from build123d import *

# Parameters (mm, degrees)
SKETCH1_W           = 4.2
SKETCH1_H           = 4.3
BOSS_EXTRUDE1_DEPTH = 7
FILLET1_R           = 1
FILLET2_R           = 3
FILLET3_R           = 1
SKETCH3_W           = 8
SKETCH3_H           = 7
BOSS_EXTRUDE2_DEPTH = 2
SKETCH2_R           = 1.4
CUT_EXTRUDE2_DEPTH  = 4
FILLET4_R           = 1


with BuildPart() as part:
    # Sketch1 → Boss-Extrude1 (new body)
    # profile 1 of 2: a face of its own
    with BuildSketch(Plane(origin=(0, 0, 0), x_dir=(1, 0, 0), z_dir=(0, 1, 0))):
        with BuildLine():
            ThreePointArc((7, 0), (-4.949747468, -4.949747468), (0, 7))
            Line((0, 7), (3.872983346, 7))
            Line((3.872983346, 7), (4, 7))
            Line((4, 7), (4, 14))
            Line((4, 14), (-4, 14))
            Line((-4, 14), (-4, 7))
            Line((-4, 7), (-3.872983346, 7))
            ThreePointArc((-3.872983346, 7), (-3.936655355, 6.964391188), (-4, 6.92820323))
            ThreePointArc((-4, 6.92820323), (-2.053343481, -7.73199719), (6.910323964, 4.030809189))
            Line((6.910323964, 4.030809189), (6.046533468, 3.52695804))
            ThreePointArc((6.046533468, 3.52695804), (6.757430513, 1.826782105), (7, 0))
        make_face()
        with Locations((0, 10.5)):
            Rectangle(SKETCH1_W, SKETCH1_H, mode=Mode.SUBTRACT)
    # profile 2 of 2: a face of its own
    with BuildSketch(Plane(origin=(0, 0, 0), x_dir=(1, 0, 0), z_dir=(0, 1, 0))):
        with BuildLine():
            Line((-4, 7), (-4, 6.92820323))
            ThreePointArc((-4, 6.92820323), (-3.936655355, 6.964391188), (-3.872983346, 7))
            Line((-3.872983346, 7), (-4, 7))
        make_face()
    extrude(amount=BOSS_EXTRUDE1_DEPTH)

    # Fillet1
    fillet1_edges = [part.edges().sort_by_distance(p)[0] for p in [
        (4, 3.5, -7),
        (-4, 3.5, -6.92820323),
    ]]
    fillet(fillet1_edges, radius=FILLET1_R)

    # Fillet2
    fillet2_edges = [part.edges().sort_by_distance(p)[0] for p in [
        (6.478428716, 0, -3.778883614),
        (6.478428716, 7, -3.778883614),
    ]]
    fillet(fillet2_edges, radius=FILLET2_R)

    # Fillet3
    fillet3_edges = [part.edges().sort_by_distance(p)[0] for p in [
        (0, 7, -8.35),
        (0, 0, -8.35),
    ]]
    fillet(fillet3_edges, radius=FILLET3_R)

    # Sketch3 → Boss-Extrude2 (add)
    with BuildSketch(Plane(origin=(0, 0, -14), x_dir=(-1, 0, 0), z_dir=(0, 0, -1))):
        with Locations((0, 3.5)):
            Rectangle(SKETCH3_W, SKETCH3_H)
    extrude(amount=BOSS_EXTRUDE2_DEPTH)

    # Sketch2 → Cut-Extrude2 (cut)
    with BuildSketch(Plane(origin=(0, 0, -16), x_dir=(-1, 0, 0), z_dir=(0, 0, -1))):
        with Locations((0, 3.5)):
            Circle(SKETCH2_R)
    extrude(amount=-CUT_EXTRUDE2_DEPTH, mode=Mode.SUBTRACT)

    # Fillet4
    fillet4_edges = [part.edges().sort_by_distance(p)[0] for p in [
        (4, 3.5, -16),
        (-4, 3.5, -16),
    ]]
    fillet(fillet4_edges, radius=FILLET4_R)


solid = part.part
Source: CAD feature listing. Evaluate the final solid. Frame: model axes, mm. A direction names the side the tool comes from. Give positions to 0.01 mm unless a question says otherwise; leave off trailing zeros. Write each loop counter-clockwise with the first axis right and the second up, starting at its lowest first coordinate (ties: lowest second). Pieces come first, ordered by that corner, then holes. Notation, with made-up numbers: (28, -31.5) -> (84, -31.5) arc R4 ccw to (84, -27.5) -> close; hole circle Ø4 at (-39.5, 64.25). An arc over 180 degrees is marked (long way). Return JSON: item names as keys, results as strings. Group by question number.
1. Material intervals for line 1 (Y direction, x = 0, z = -14.15); line 2 (X direction, y = 5, z = -11.25); line 3 (Z direction, x = 0, y = 3.25), sorted ascending. Write a range as from..to.
2. Section C-C, the plane z = 6. Output: boundary loops of the cut face in (x, y), then the cut area to 3 significant figures.
3. Access query for faces 1 (the face through (6.48, 3.49, -3.78)), 2 (the face through (3.715, 3.549, -7.301)), 3 (the face through (4, 3, -11)), 4 (the face through (0.303, 2.133, -14.348)). Directions: +Z, -Z, +X, -X, +Y, -Y. A direction counts if a zero-diameter tool reaches every point of the face in a straight line with its end or side. Return the directions, or none.
4. Pin query (flat end, axial travel): pin 1 Ø1 at (y, z) = (2.5, -8.5) entering from -X; pin 2 Ø0.9 at (x, y) = (2, 5) entering from +Z; pin 3 Ø2 at (y, z) = (2.5, -12.5) entering from +X. Return the tip coordinate at first contact, or that it passes through.
5. Section B-B, the plane y = 3.5. Output: boundary loops of the cut face in (x, z), then the cut area to 3 significant figures.
6. Section A-A, the plane x = -3.5. Output: boundary loops of the cut face in (y, z).
7. Section D-D, the plane x = 0.25. Output: boundary loops of the cut face in (y, z), then the cut area to 3 significant figures.
8. Mould query, pull axis Z, two halves, no side actions, for faces 5 (the face through (-2, 0, -7)), 6 (the face through (6.79, 6.14, -2.92)), 7 (the face through (0.029, 6.699, -8.065)). Classes: +Z half, -Z half, draft (parallel to the pull), parting line (faces both ways), or undercut.
Determined:
{
 "1": {"line 1": "y = 0..2.1, 4.9..7", "line 2": "x = -4..-2.1, 2.1..4", "line 3": "z = -8.35..-7, 7..8"},
 "2": {"outline": "(-5.29, 0) -> (-3.61, 0) -> (-3.61, 7) -> (-5.29, 7) -> close; (3.61, 0) -> (5.29, 0) -> (5.29, 7) -> (3.61, 7) -> close", "area": "23.6 mm2"},
 "3": {"face 1": "-Z, +Y, -Y", "face 2": "+X, +Y, -Y", "face 3": "-Z, +X, +Y, -Y", "face 4": "-Z"},
 "4": {"pin 1": "stops at x = -4", "pin 2": "stops at z = 7.85", "pin 3": "stops at x = 4"},
 "5": {"outline": "(-4.44, -6.65) arc R1 cw to (-4, -7.48) -> (-4, -15) arc R1 ccw to (-3, -16) -> (-1.4, -16) -> (-1.4, -12.65) -> (-2.1, -12.65) -> (-2.1, -8.35) -> (2.1, -8.35) -> (2.1, -12.65) -> (1.4, -12.65) -> (1.4, -16) -> (3, -16) arc R1 ccw to (4, -15) -> (4, -8) arc R1 ccw to (3, -7) -> (0, -7) arc R7 cw (long way) to (6.05, -3.53) -> (6.91, -4.03) arc R8 ccw (long way) to start", "area": "80.7 mm2"},
 "6": {"outline": "(0, -15.87) -> (7, -15.87) -> (7, -6.06) -> (0, -6.06) -> close; (0, 6.06) -> (7, 6.06) -> (7, 7.19) -> (0, 7.19) -> close"},
 "7": {"outline": "(0, -16) -> (2.12, -16) -> (2.12, -12.65) -> (0, -12.65) -> close; (0, -7.35) arc R1 ccw to (1, -8.35) -> (6, -8.35) arc R1 ccw to (7, -7.35) -> (7, -7) -> (0, -7) -> close; (0, 7) -> (7, 7) -> (7, 8) -> (0, 8) -> close; (4.88, -16) -> (7, -16) -> (7, -12.65) -> (4.88, -12.65) -> close", "area": "30.2 mm2"},
 "8": {"face 5": "draft", "face 6": "-Z half", "face 7": "undercut"}
}
